For this review, take the finished solid that the model builds, in its own axes (mm). A direction names the side the tool comes from. Round coordinates to 2 decimals unless told otherwise and drop trailing zeros. Loops run counter-clockwise (first coordinate to the right, second up) from the corner with the lowest first, then second, coordinate; pieces in that order, holes last.
```python
from build123d import *

# Parameters (mm, degrees)
F0_R     = 5.1978501012
F1_DEPTH = 2.54


with BuildPart() as f1:
    # F0 (on Top) → F1 (new body)
    with BuildSketch(Plane.XY):
        with BuildLine():
            Line((36.8412211885, 14.7556602153), (-39.3587788115, 14.7556602153))
            ThreePointArc((-39.3587788115, 14.7556602153), (-52.0587788115, 2.0556602153), (-39.3587788115, -10.6443397847))
            Line((-39.3587788115, -10.6443397847), (36.8412211885, -10.6443397847))
            Line((36.8412211885, -10.6443397847), (36.8412211885, 14.7556602153))
        make_face()
        with Locations((-44.5566289127, 2.0556602153)):
            Circle(F0_R, mode=Mode.SUBTRACT)
        with BuildLine():
            add(Edge.make_bspline(
                [(-22.306449124, 1.1279649028), (-21.5209673532, 0.1109727153), (-21.5209673532, -1.3673866597)],
                knots=[0, 0, 0, 1, 1, 1], degree=2))
            add(Edge.make_bspline(
                [(-21.5209673532, -1.3673866597), (-21.5209673532, -3.4146002013), (-22.9943657907, -4.5936496805)],
                knots=[0, 0, 0, 1, 1, 1], degree=2))
            add(Edge.make_bspline(
                [(-22.9943657907, -4.5936496805), (-24.4677642282, -5.7726991597), (-27.0904465199, -5.7726991597)],
                knots=[0, 0, 0, 1, 1, 1], degree=2))
            add(Edge.make_bspline(
                [(-27.0904465199, -5.7726991597), (-29.5113840199, -5.7726991597), (-31.3700819365, -4.8598866597)],
                knots=[0, 0, 0, 1, 1, 1], degree=2))
            Line((-31.3700819365, -4.8598866597), (-31.3700819365, -1.8833241597))
            add(Edge.make_bspline(
                [(-31.3700819365, -1.8833241597), (-29.8421131865, -2.5679335347), (-28.7821262074, -2.8457460347)],
                knots=[0, 0, 0, 1, 1, 1], degree=2))
            add(Edge.make_bspline(
                [(-28.7821262074, -2.8457460347), (-27.7221392282, -3.1235585347), (-26.8423996449, -3.1235585347)],
                knots=[0, 0, 0, 1, 1, 1], degree=2))
            add(Edge.make_bspline(
                [(-26.8423996449, -3.1235585347), (-25.7906808949, -3.1235585347), (-25.2267876657, -2.7217225972)],
                knots=[0, 0, 0, 1, 1, 1], degree=2))
            add(Edge.make_bspline(
                [(-25.2267876657, -2.7217225972), (-24.6628944365, -2.3198866597), (-24.6628944365, -1.522829368)],
                knots=[0, 0, 0, 1, 1, 1], degree=2))
            add(Edge.make_bspline(
                [(-24.6628944365, -1.522829368), (-24.6628944365, -1.0796522847), (-24.9109413115, -0.7323866597)],
                knots=[0, 0, 0, 1, 1, 1], degree=2))
            add(Edge.make_bspline(
                [(-24.9109413115, -0.7323866597), (-25.1589881865, -0.3851210347), (-25.640199124, -0.0659673888)],
                knots=[0, 0, 0, 1, 1, 1], degree=2))
            add(Edge.make_bspline(
                [(-25.640199124, -0.0659673888), (-26.1214100615, 0.253186257), (-27.5997694365, 0.957639382)],
                knots=[0, 0, 0, 1, 1, 1], degree=2))
            add(Edge.make_bspline(
                [(-27.5997694365, 0.957639382), (-28.9822173532, 1.6091758403), (-29.6750949574, 2.207795632)],
                knots=[0, 0, 0, 1, 1, 1], degree=2))
            add(Edge.make_bspline(
                [(-29.6750949574, 2.207795632), (-30.3679725615, 2.8064154237), (-30.7813840199, 3.6034727153)],
                knots=[0, 0, 0, 1, 1, 1], degree=2))
            add(Edge.make_bspline(
                [(-30.7813840199, 3.6034727153), (-31.1947954782, 4.400530007), (-31.1947954782, 5.462170632)],
                knots=[0, 0, 0, 1, 1, 1], degree=2))
            add(Edge.make_bspline(
                [(-31.1947954782, 5.462170632), (-31.1947954782, 7.4696966737), (-29.8354986032, 8.6156732362)],
                knots=[0, 0, 0, 1, 1, 1], degree=2))
            add(Edge.make_bspline(
                [(-29.8354986032, 8.6156732362), (-28.4762017282, 9.7616497987), (-26.0784152699, 9.7616497987)],
                knots=[0, 0, 0, 1, 1, 1], degree=2))
            add(Edge.make_bspline(
                [(-26.0784152699, 9.7616497987), (-24.9010194365, 9.7616497987), (-23.8311105824, 9.4838372987)],
                knots=[0, 0, 0, 1, 1, 1], degree=2))
            add(Edge.make_bspline(
                [(-23.8311105824, 9.4838372987), (-22.7612017282, 9.2060247987), (-21.5937277699, 8.7000091737)],
                knots=[0, 0, 0, 1, 1, 1], degree=2))
            Line((-21.5937277699, 8.7000091737), (-22.6256027699, 6.206311257))
            add(Edge.make_bspline(
                [(-22.6256027699, 6.206311257), (-23.8360715199, 6.702405007), (-24.6265142282, 6.8991888612)],
                knots=[0, 0, 0, 1, 1, 1], degree=2))
            add(Edge.make_bspline(
                [(-24.6265142282, 6.8991888612), (-25.4169569365, 7.0959727153), (-26.1809413115, 7.0959727153)],
                knots=[0, 0, 0, 1, 1, 1], degree=2))
            add(Edge.make_bspline(
                [(-26.1809413115, 7.0959727153), (-27.0904465199, 7.0959727153), (-27.5766183949, 6.672639382)],
                knots=[0, 0, 0, 1, 1, 1], degree=2))
            add(Edge.make_bspline(
                [(-27.5766183949, 6.672639382), (-28.0627902699, 6.2493060487), (-28.0627902699, 5.5680039653)],
                knots=[0, 0, 0, 1, 1, 1], degree=2))
            add(Edge.make_bspline(
                [(-28.0627902699, 5.5680039653), (-28.0627902699, 5.144670632), (-27.8660064157, 4.8288242778)],
                knots=[0, 0, 0, 1, 1, 1], degree=2))
            add(Edge.make_bspline(
                [(-27.8660064157, 4.8288242778), (-27.6692225615, 4.5129779237), (-27.2409282907, 4.2186289653)],
                knots=[0, 0, 0, 1, 1, 1], degree=2))
            add(Edge.make_bspline(
                [(-27.2409282907, 4.2186289653), (-26.8126340199, 3.924280007), (-25.2119048532, 3.160295632)],
                knots=[0, 0, 0, 1, 1, 1], degree=2))
            add(Edge.make_bspline(
                [(-25.2119048532, 3.160295632), (-23.0919308949, 2.1449570903), (-22.306449124, 1.1279649028)],
                knots=[0, 0, 0, 1, 1, 1], degree=2))
        make_face(mode=Mode.SUBTRACT)
        with BuildLine():
            Line((-13.0245350615, 0.5541497987), (-10.1637277699, 9.5466758403))
            Line((-10.1637277699, 9.5466758403), (-6.9291965199, 9.5466758403))
            Line((-6.9291965199, 9.5466758403), (-12.0654204782, -5.5643397847))
            Line((-12.0654204782, -5.5643397847), (-15.5579204782, -5.5643397847))
            Line((-15.5579204782, -5.5643397847), (-20.6842225615, 9.5466758403))
            Line((-20.6842225615, 9.5466758403), (-17.4496913115, 9.5466758403))
            Line((-17.4496913115, 9.5466758403), (-14.6054204782, 0.5541497987))
            add(Edge.make_bspline(
                [(-14.6054204782, 0.5541497987), (-14.3706027699, -0.242907493), (-14.1159413115, -1.3012408263)],
                knots=[0, 0, 0, 1, 1, 1], degree=2))
            add(Edge.make_bspline(
                [(-14.1159413115, -1.3012408263), (-13.8612798532, -2.3595741597), (-13.8017486032, -2.772985618)],
                knots=[0, 0, 0, 1, 1, 1], degree=2))
            add(Edge.make_bspline(
                [(-13.8017486032, -2.772985618), (-13.6859933949, -1.8237929097), (-13.0245350615, 0.5541497987)],
                knots=[0, 0, 0, 1, 1, 1], degree=2))
        make_face(mode=Mode.SUBTRACT)
        Polygon((3.6739805635, -2.9185064513), (3.6739805635, -5.5643397847), (-5.0275038115, -5.5643397847), (-5.0275038115, 9.5466758403), (3.6739805635, 9.5466758403), (3.6739805635, 6.920686257), (-1.8227381865, 6.920686257), (-1.8227381865, 3.6034727153), (3.2936420218, 3.6034727153), (3.2936420218, 0.977483132), (-1.8227381865, 0.977483132), (-1.8227381865, -2.9185064513), align=None, mode=Mode.SUBTRACT)
        with BuildLine():
            add(Edge.make_bspline(
                [(14.960113376, 1.1279649028), (15.7455951468, 0.1109727153), (15.7455951468, -1.3673866597)],
                knots=[0, 0, 0, 1, 1, 1], degree=2))
            add(Edge.make_bspline(
                [(15.7455951468, -1.3673866597), (15.7455951468, -3.4146002013), (14.2721967093, -4.5936496805)],
                knots=[0, 0, 0, 1, 1, 1], degree=2))
            add(Edge.make_bspline(
                [(14.2721967093, -4.5936496805), (12.7987982718, -5.7726991597), (10.1761159801, -5.7726991597)],
                knots=[0, 0, 0, 1, 1, 1], degree=2))
            add(Edge.make_bspline(
                [(10.1761159801, -5.7726991597), (7.7551784801, -5.7726991597), (5.8964805635, -4.8598866597)],
                knots=[0, 0, 0, 1, 1, 1], degree=2))
            Line((5.8964805635, -4.8598866597), (5.8964805635, -1.8833241597))
            add(Edge.make_bspline(
                [(5.8964805635, -1.8833241597), (7.4244493135, -2.5679335347), (8.4844362926, -2.8457460347)],
                knots=[0, 0, 0, 1, 1, 1], degree=2))
            add(Edge.make_bspline(
                [(8.4844362926, -2.8457460347), (9.5444232718, -3.1235585347), (10.4241628551, -3.1235585347)],
                knots=[0, 0, 0, 1, 1, 1], degree=2))
            add(Edge.make_bspline(
                [(10.4241628551, -3.1235585347), (11.4758816051, -3.1235585347), (12.0397748343, -2.7217225972)],
                knots=[0, 0, 0, 1, 1, 1], degree=2))
            add(Edge.make_bspline(
                [(12.0397748343, -2.7217225972), (12.6036680635, -2.3198866597), (12.6036680635, -1.522829368)],
                knots=[0, 0, 0, 1, 1, 1], degree=2))
            add(Edge.make_bspline(
                [(12.6036680635, -1.522829368), (12.6036680635, -1.0796522847), (12.3556211885, -0.7323866597)],
                knots=[0, 0, 0, 1, 1, 1], degree=2))
            add(Edge.make_bspline(
                [(12.3556211885, -0.7323866597), (12.1075743135, -0.3851210347), (11.626363376, -0.0659673888)],
                knots=[0, 0, 0, 1, 1, 1], degree=2))
            add(Edge.make_bspline(
                [(11.626363376, -0.0659673888), (11.1451524385, 0.253186257), (9.6667930635, 0.957639382)],
                knots=[0, 0, 0, 1, 1, 1], degree=2))
            add(Edge.make_bspline(
                [(9.6667930635, 0.957639382), (8.2843451468, 1.6091758403), (7.5914675426, 2.207795632)],
                knots=[0, 0, 0, 1, 1, 1], degree=2))
            add(Edge.make_bspline(
                [(7.5914675426, 2.207795632), (6.8985899385, 2.8064154237), (6.4851784801, 3.6034727153)],
                knots=[0, 0, 0, 1, 1, 1], degree=2))
            add(Edge.make_bspline(
                [(6.4851784801, 3.6034727153), (6.0717670218, 4.400530007), (6.0717670218, 5.462170632)],
                knots=[0, 0, 0, 1, 1, 1], degree=2))
            add(Edge.make_bspline(
                [(6.0717670218, 5.462170632), (6.0717670218, 7.4696966737), (7.4310638968, 8.6156732362)],
                knots=[0, 0, 0, 1, 1, 1], degree=2))
            add(Edge.make_bspline(
                [(7.4310638968, 8.6156732362), (8.7903607718, 9.7616497987), (11.1881472301, 9.7616497987)],
                knots=[0, 0, 0, 1, 1, 1], degree=2))
            add(Edge.make_bspline(
                [(11.1881472301, 9.7616497987), (12.3655430635, 9.7616497987), (13.4354519176, 9.4838372987)],
                knots=[0, 0, 0, 1, 1, 1], degree=2))
            add(Edge.make_bspline(
                [(13.4354519176, 9.4838372987), (14.5053607718, 9.2060247987), (15.6728347301, 8.7000091737)],
                knots=[0, 0, 0, 1, 1, 1], degree=2))
            Line((15.6728347301, 8.7000091737), (14.6409597301, 6.206311257))
            add(Edge.make_bspline(
                [(14.6409597301, 6.206311257), (13.4304909801, 6.702405007), (12.6400482718, 6.8991888612)],
                knots=[0, 0, 0, 1, 1, 1], degree=2))
            add(Edge.make_bspline(
                [(12.6400482718, 6.8991888612), (11.8496055635, 7.0959727153), (11.0856211885, 7.0959727153)],
                knots=[0, 0, 0, 1, 1, 1], degree=2))
            add(Edge.make_bspline(
                [(11.0856211885, 7.0959727153), (10.1761159801, 7.0959727153), (9.6899441051, 6.672639382)],
                knots=[0, 0, 0, 1, 1, 1], degree=2))
            add(Edge.make_bspline(
                [(9.6899441051, 6.672639382), (9.2037722301, 6.2493060487), (9.2037722301, 5.5680039653)],
                knots=[0, 0, 0, 1, 1, 1], degree=2))
            add(Edge.make_bspline(
                [(9.2037722301, 5.5680039653), (9.2037722301, 5.144670632), (9.4005560843, 4.8288242778)],
                knots=[0, 0, 0, 1, 1, 1], degree=2))
            add(Edge.make_bspline(
                [(9.4005560843, 4.8288242778), (9.5973399385, 4.5129779237), (10.0256342093, 4.2186289653)],
                knots=[0, 0, 0, 1, 1, 1], degree=2))
            add(Edge.make_bspline(
                [(10.0256342093, 4.2186289653), (10.4539284801, 3.924280007), (12.0546576468, 3.160295632)],
                knots=[0, 0, 0, 1, 1, 1], degree=2))
            add(Edge.make_bspline(
                [(12.0546576468, 3.160295632), (14.1746316051, 2.1449570903), (14.960113376, 1.1279649028)],
                knots=[0, 0, 0, 1, 1, 1], degree=2))
        make_face(mode=Mode.SUBTRACT)
    extrude(amount=F1_DEPTH)


solid = f1.part
```
(1) The part is to be moulded in two halves that separate along X. For faces 3 (the flat face through (-8, 2, 2.54)), 4 (the flat face through (-1.823, 5, 1)), 5 (the cylindrical face through (-52.056, 2.335, 1.252)), say which applies: pulls with the +X half, pulls with the -X half, needs draft (parallel to the pull), parting line crosses it, or undercut.
(2) For L1, parallel to Y at x = 1.5, z = 2.1; L2, parallel to X at y = 7.5, z = 2.1; L3, parallel to Y at x = 7.5, z = 2.2, list the stretches that pass through material, from the lowest coordinate up.
(3) Add section B-B (z = 0.85). Give the number of separate pieces and of enclosed holes in the cut face, plus the area to 3 significant figures.
(4) For faces 1 (the flat face through (3.674, -4, 1)), 2 (the flat face through (36.841, 2, 1)), list the 3-axis set-ups (+Z, -Z, +X, -X, +Y, -Y) from which the entire face can be reached by the end or side of a thin tool; tool diameter is ignored.
(5) Add section A-A (x = -44.5). Give the boundary of the cut face in (y, z).
(6) Insertion check: pin 1 Ø0.8 at (y, z) = (-1.5, 2) entering from -X; pin 2 Ø1.3 at (y, z) = (8.5, 1.5) entering from -X. Each pin has a flat end and moves straight along its axis. Give the tip position at first contact, or say it passes through.
Outcome:
1. face 3: needs draft
1. face 4: undercut
1. face 5: pulls with the -X half
2. L1: y = -10.64 to -5.56, -2.92 to 0.98, 3.6 to 6.92, 9.55 to 14.76
2. L2: x = -50.83 to -30.74, -22.09 to -19.99, -16.8 to -10.81, -7.62 to -5.03, 3.67 to 6.53, 15.18 to 36.84
2. L3: y = -10.64 to -5.45, -2.54 to 2.29, 8.67 to 14.76
3. separate pieces: 1
3. enclosed holes: 5
3. area: 1,750 mm2
4. face 1: +Z, -Z
4. face 2: +Z, -Z, +X, +Y, -Y
5. outline: (-9.56, 0) - (-3.14, 0) - (-3.14, 2.54) - (-9.56, 2.54) - close; (7.25, 0) - (13.67, 0) - (13.67, 2.54) - (7.25, 2.54) - close
6. pin 1: stops at x = -51.66
6. pin 2: stops at x = -50.66
